Here's how the part is built. I have some questions about the finished solid (model axes, mm). A direction names the side the tool comes from. Round coordinates to 2 decimals unless told otherwise and drop trailing zeros. Write each loop counter-clockwise with the first axis right and the second up, starting at its lowest first coordinate (ties: lowest second). Pieces come first, ordered by that corner, then holes. Notation, with made-up numbers: (7.5, 21) - (13.5, 21) arc R21 cw to (13.5, 34) - close; hole circle Ø6 at (-19, -29.5). An arc over 180 degrees is marked (long way). One line per question, with ' | ' between items. Start each with the question number.
(1) For faces 1 (the cylindrical face through (54.93, 122.87, 36.5)), 2 (the flat face through (-1, 104, 0)), 3 (the flat face through (0.49, 157.08, 59.26)), which set-ups out of +Z, -Z, +X, -X, +Y, -Y let a thin tool reach every point of the face, with its end or its side?
(2) Imagine slicing it at C-C (z = 83). Write out the boundary of the cut face in (x, y), plus the area to 3 significant figures.
(3) Imagine slicing it at B-B (z = 39.1). Write out the boundary of the cut face in (x, y), plus the area to 3 significant figures.
(4) Thinking about a two-plate mould opening in X: for faces 4 (the cylindrical face through (5.77, 157.686, 39.76)), 5 (the flat face through (-50, 124, 27)), 6 (the cylindrical face through (40, 20, 17)), which applies, pulls with the +X half, pulls with the -X half, needs draft (parallel to the pull), parting line crosses it, or undercut?
(5) If I drill on L1, parallel to Y at x = 9, z = 39.1; L2, parallel to X at y = 115, z = 45; L3, parallel to Z at x = 20, y = 65, over which ranges is the centre line in solid material (lowest first)?
(6) Imagine slicing it at A-A (x = -42). Write out the boundary of the cut face in (y, z).
(7) Imagine slicing it at D-D (y = 86). Write out the boundary of the cut face in (x, z), plus the area to 3 significant figures.
(8) Will these pins go through, and if not, where does the flat tip stop? pin 1 (10 mm diameter, centred on x = 43, z = 85, fed in from -Y); pin 2 (4 mm diameter, centred on x = 30.5, z = 63.5, fed in from +Y); pin 3 (24 mm diameter, centred on x = -23, z = 55, fed in from -Y).
from build123d import *

# Parameters (mm, degrees)
EXTRUDE_1_DEPTH          = 34.1
FILLET_2_R               = 20
SKETCH_1_5_W             = 50
SKETCH_1_5_H             = 84.9
EXTRUDE_3_DEPTH          = 34.1
SKETCH_4_W               = 20
SKETCH_4_H               = 20
EXTRUDE_4_DEPTH          = 50
EXTRUDE_5_DEPTH          = 50
SKETCH_7_R               = 15
CUT_EXTRUDE_1_DEPTH      = 219.119470794
SKETCH_8_W               = 35
SKETCH_8_H               = 15
CUT_EXTRUDE_2_DEPTH      = 212.953207538
FILLET_2_OF_MIRROR_1_R   = 20
SKETCH_13_R              = 20
EXTRUDE_6_DEPTH          = 10
CUT_EXTRUDE_3_DEPTH      = 235.682985193
CUT_EXTRUDE_3_DEPTH_BACK = 235.682985193
SKETCH_15_R              = 15


with BuildPart() as part:
    # Эскиз1 → Бобышка-Вытянуть1 (new body)
    with BuildSketch(Plane.XY):
        with BuildLine():
            ThreePointArc((30, 10), (40, 20), (30, 30))
            Line((30, 30), (0, 30))
            Line((0, 30), (0, 102.653608526))
            Line((0, 102.653608526), (50, 102.653608526))
            Line((50, 102.653608526), (50, 82.653608526))
            ThreePointArc((50, 82.653608526), (30, 62.653608526), (50, 42.653608526))
            Line((50, 42.653608526), (50, 0))
            Line((50, 0), (0, 0))
            Line((0, 0), (0, 10))
            Line((0, 10), (30, 10))
        make_face()
    extrude_1 = extrude(amount=EXTRUDE_1_DEPTH)

    # Скругление2
    fillet_2_edges = [part.edges().sort_by_distance(p)[0] for p in [
        (50, 0, 17.05),
    ]]
    fillet(fillet_2_edges, radius=FILLET_2_R)

    # Эскиз1<5> → Бобышка-Вытянуть3 (add)
    with BuildSketch(Plane.XY):
        with Locations((25, 145.103608526)):
            Rectangle(SKETCH_1_5_W, SKETCH_1_5_H)
    extrude_3 = extrude(amount=EXTRUDE_3_DEPTH)

    # Эскиз4 → Бобышка-Вытянуть4 (add)
    with BuildSketch(Plane(origin=(50, 0, 0), x_dir=(0, 0, -1), z_dir=(1, 0, 0))):
        with Locations((10, 177.553608526)):
            Rectangle(SKETCH_4_W, SKETCH_4_H)
    extrude_4 = extrude(amount=-EXTRUDE_4_DEPTH)

    # Эскиз5 → Бобышка-Вытянуть5 (add)
    with BuildSketch(Plane(origin=(50, 0, 0), x_dir=(0, 0, -1), z_dir=(1, 0, 0))):
        Polygon((-34.1, 187.553608526), (-50, 187.553608526), (-99.497474683, 138.056133842), (-64.142135624, 102.700794783), (-34.1, 102.700794783), align=None)
    extrude_5 = extrude(amount=-EXTRUDE_5_DEPTH)

    # Эскиз7 → Вырез-Вытянуть1 (cut, symmetric)
    with BuildSketch(Plane(origin=(50, 0, 0), x_dir=(0, 0, -1), z_dir=(1, 0, 0))):
        with Locations((-39.1, 142.700794783)):
            Circle(SKETCH_7_R)
    cut_extrude_1 = extrude(amount=CUT_EXTRUDE_1_DEPTH, both=True, mode=Mode.SUBTRACT)

    # Эскиз8 → Вырез-Вытянуть2 (cut, through all)
    with BuildSketch(Plane(origin=(0, 19.27932958, -19.27932958), x_dir=(1, 0, 0), z_dir=(0, -0.7071067811865498, 0.7071067811865454))):
        with Locations((17.5, 160.475767484)):
            Rectangle(SKETCH_8_W, SKETCH_8_H)
    cut_extrude_2 = extrude(amount=-CUT_EXTRUDE_2_DEPTH, mode=Mode.SUBTRACT)

    # Зеркальное отражение1: Бобышка-Вытянуть1, Бобышка-Вытянуть3, Бобышка-Вытянуть4, Бобышка-Вытянуть5, Вырез-Вытянуть1, Вырез-Вытянуть2 across plane
    add(extrude_1.mirror(Plane(origin=(0, 0, 34.1), x_dir=(0, 0, 1), z_dir=(1, 0, 0))))
    add(extrude_3.mirror(Plane(origin=(0, 0, 34.1), x_dir=(0, 0, 1), z_dir=(1, 0, 0))))
    add(extrude_4.mirror(Plane(origin=(0, 0, 34.1), x_dir=(0, 0, 1), z_dir=(1, 0, 0))))
    add(extrude_5.mirror(Plane(origin=(0, 0, 34.1), x_dir=(0, 0, 1), z_dir=(1, 0, 0))))
    add(cut_extrude_1.mirror(Plane(origin=(0, 0, 34.1), x_dir=(0, 0, 1), z_dir=(1, 0, 0))), mode=Mode.SUBTRACT)
    add(cut_extrude_2.mirror(Plane(origin=(0, 0, 34.1), x_dir=(0, 0, 1), z_dir=(1, 0, 0))), mode=Mode.SUBTRACT)

    # Скругление2 of Зеркальное отражение1
    fillet_2_of_mirror_1_edges = [part.edges().sort_by_distance(p)[0] for p in [
        (-50, 0, 17.05),
    ]]
    fillet(fillet_2_of_mirror_1_edges, radius=FILLET_2_OF_MIRROR_1_R)

    # Эскиз13 → Бобышка-Вытянуть6 (add)
    with BuildSketch(Plane(origin=(50, 0, 0), x_dir=(0, 0, -1), z_dir=(1, 0, 0))):
        with Locations(Location((-39.1, 142.700794783, 0), (0, 0, 180))):
            Circle(SKETCH_13_R)
    extrude(amount=EXTRUDE_6_DEPTH)

    # Эскиз15 → Вырез-Вытянуть3 (cut, two sides: drawn at the far end of the back side and taken through both)
    with BuildSketch(Plane.ZY.offset(-50).offset(-CUT_EXTRUDE_3_DEPTH_BACK)):
        with Locations(Location((39.1, 142.700794783, 0), (0, 0, 270))):
            Circle(SKETCH_15_R)
    extrude(amount=CUT_EXTRUDE_3_DEPTH + CUT_EXTRUDE_3_DEPTH_BACK, mode=Mode.SUBTRACT)


solid = part.part
Check sheet entries:
1) face 1: +X | face 2: -Z, +X, -X, -Y | face 3: +Z, +Y
2) outline: (-50, 121.56) - (50, 121.56) - (50, 154.55) - (35, 154.55) - (35, 133.34) - (-35, 133.34) - (-35, 154.55) - (-50, 154.55) - close | area: 1,810 mm^2
3) outline: (-50, 102.7) - (50, 102.7) - (50, 122.7) - (60, 122.7) - (60, 127.7) - (-50, 127.7) - close; (-50, 157.7) - (60, 157.7) - (60, 162.7) - (50, 162.7) - (50, 187.55) - (35, 187.55) - (35, 177.24) - (-35, 177.24) - (-35, 187.55) - (-50, 187.55) - close | area: 4,860 mm^2
4) face 4: needs draft | face 5: pulls with the -X half | face 6: undercut
5) L1: 102.7 to 127.7, 157.7 to 177.24 | L2: -50 to 50 | L3: 0 to 34.1
6) outline: (4, 0) - (44.32, 0) - (44.32, 34.1) - (4, 34.1) - close; (80.98, 0) - (167.55, 0) - (167.55, -20) - (187.55, -20) - (187.55, 50) - (138.06, 99.5) - (102.7, 64.14) - (102.7, 34.1) - (80.98, 34.1) - close; hole circle Ø30 at (142.7, 39.1)
7) outline: (-50, 0) - (50, 0) - (50, 34.1) - (-50, 34.1) - close | area: 3,410 mm^2
8) pin 1: y = 118.56 | pin 2: y = 154.84 | pin 3: y = 102.7
